Design review of the part built by this model. Coordinates are the model's own, in mm. Face numbers are marked on the shaded views. A direction names the side the tool comes from. Round coordinates to 2 decimals unless told otherwise and drop trailing zeros. Order: outer loops, then holes, each group sorted by start corner. A loop starts at its lowest first (then second) coordinate and runs counter-clockwise, first axis right, second up. Notation, with made-up numbers: (-30.5, 51.25) - (-14.5, 51.25) arc R14 ccw to (-14.5, 68.25) - close; hole circle Ø3 at (80.25, 27.25). An arc over 180 degrees is marked (long way). Answer as a JSON object with one key per item and string values. Group by question number.
from build123d import *

# Parameters (mm, degrees)
F0_W      = 1270
F0_H      = 660.4
F1_DEPTH  = 101.6
F2_W      = 101.6
F2_H      = 101.6
F3_DEPTH  = 304.8
F4_W      = 101.6
F4_H      = 101.6
F5_DEPTH  = 304.8
F6_DEPTH  = 304.8
F8_W      = 101.6
F8_H      = 101.6
F9_DEPTH  = 304.8
F7_W      = 101.6
F7_H      = 101.6
F10_DEPTH = 304.8


with BuildPart() as f1:
    # F0 (on Front) → F1 (new body)
    with BuildSketch(Plane.XZ):
        Rectangle(F0_W, F0_H)
        Polygon((533.4, 173.331247), (533.4, -228.6), (-404.439575, -228.6), (-533.4, -228.6), (-533.4, -173.331247), (-533.4, 228.6), (404.439575, 228.6), (533.4, 228.6), align=None, mode=Mode.SUBTRACT)
        Polygon((-533.4, -228.6), (-404.439575, -228.6), (533.4, 173.331247), (533.4, 228.6), (404.439575, 228.6), (-533.4, -173.331247), align=None)
    extrude(amount=F1_DEPTH)

    # F2 (on face) → F3 (join)
    with BuildSketch(Plane.XZ.offset(101.6)):
        with Locations((-584.2, 279.4)):
            Rectangle(F2_W, F2_H)
    extrude(amount=F3_DEPTH)

    # F4 (on face) → F5 (join)
    with BuildSketch(Plane.XZ.offset(101.6)):
        with Locations((-584.2, -279.4)):
            Rectangle(F4_W, F4_H)
    extrude(amount=F5_DEPTH)

    # F4 (on face) → F6 (join)
    with BuildSketch(Plane.XZ.offset(101.6)):
        with Locations((-584.2, -279.4)):
            Rectangle(F4_W, F4_H)
    extrude(amount=F6_DEPTH)

    # F8 (on face) → F9 (join)
    with BuildSketch(Plane.XZ.offset(101.6)):
        with Locations((584.2, 279.4)):
            Rectangle(F8_W, F8_H)
    extrude(amount=F9_DEPTH)

    # F7 (on face) → F10 (join)
    with BuildSketch(Plane.XZ.offset(101.6)):
        with Locations((584.2, -279.4)):
            Rectangle(F7_W, F7_H)
    extrude(amount=F10_DEPTH)


solid = f1.part
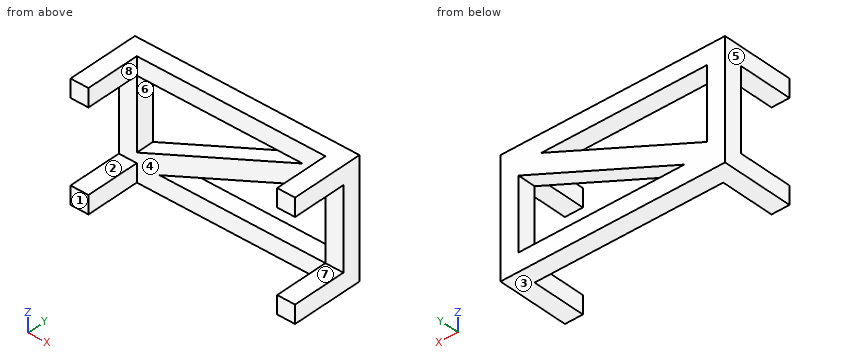
1. Tool access review of the marked faces 5, 6, 7 and 8: name each direction out of +Z, -Z, +X, -X, +Y, -Y from which nothing blocks a thin tool from reaching the whole face with its end or side.
2. Take a section at B-B, the plane x = -484. Give the boundary of the cut face in (y, z), then the cut area to 3 significant figures.
3. Take a section at A-A, the plane y = -199. Give the boundary of the cut face in (x, z).
4. Take a section at D-D, the plane y = -71. Give the boundary of the cut face in (x, z).
5. To check wall thickness, follow line 1 (X direction, y = -18, z = 14); line 2 (X direction, y = -175.5, z = -237); line 3 (Z direction, x = -8, y = -34). State the ranges of each line that lie inside material, in increasing order. Write a range as from..to.
6. Mouldability with a two-part tool opening along Z and no side actions: class the marked faces 1, 2, 3 and 4 as pulls with the +Z half, pulls with the -Z half, needs draft (parallel to the pull), parting line crosses it, or undercut.
7. Take a section at C-C, the plane z = -109.5. Give the boundary of the cut face in (x, y), then the cut area to 4 significant figures.
Response values:
{
 "1": {"face 5": "+Z, -Z, -X, +Y, -Y", "face 6": "+Y, -Y", "face 7": "+X, -X, -Y", "face 8": "+Z, -Z, -Y"},
 "2": {"outline": "(-101.6, -330.2) - (0, -330.2) - (0, -152.16) - (-101.6, -152.16) - close; (-101.6, 228.6) - (0, 228.6) - (0, 330.2) - (-101.6, 330.2) - close", "area": "28,400 mm2"},
 "3": {"outline": "(-635, -330.2) - (-533.4, -330.2) - (-533.4, -228.6) - (-635, -228.6) - close; (-635, 228.6) - (-533.4, 228.6) - (-533.4, 330.2) - (-635, 330.2) - close; (533.4, -330.2) - (635, -330.2) - (635, -228.6) - (533.4, -228.6) - close; (533.4, 228.6) - (635, 228.6) - (635, 330.2) - (533.4, 330.2) - close"},
 "4": {"outline": "(-635, -330.2) - (635, -330.2) - (635, 330.2) - (-635, 330.2) - close; hole (-533.4, -173.33) - (404.44, 228.6) - (-533.4, 228.6) - close; hole (-404.44, -228.6) - (533.4, -228.6) - (533.4, 173.33) - close"},
 "5": {"line 1": "-635..-533.4, -96.29..161.63, 533.4..635", "line 2": "-635..-533.4, 533.4..635", "line 3": "-330.2..-228.6, -58.7..51.84, 228.6..330.2"},
 "6": {"face 1": "needs draft", "face 2": "undercut", "face 3": "pulls with the -Z half", "face 4": "undercut"},
 "7": {"outline": "(-635, -101.6) - (-533.4, -101.6) - (-533.4, 0) - (-635, 0) - close; (-384.46, -101.6) - (-126.54, -101.6) - (-126.54, 0) - (-384.46, 0) - close; (533.4, -101.6) - (635, -101.6) - (635, 0) - (533.4, 0) - close", "area": "46,850 mm2"}
}
